For this review, take the finished solid that the model builds, in its own axes (mm). Give positions to 0.01 mm unless a question says otherwise; leave off trailing zeros. Loops run counter-clockwise (first coordinate to the right, second up) from the corner with the lowest first, then second, coordinate; pieces in that order, holes last. Notation, with made-up numbers: (-23.5, -3) -> (3.5, -3) arc R20 cw to (3.5, 14) -> close; hole circle Ø5 at (-4, -14.75). An arc over 180 degrees is marked (long way). Answer as CSV lines item,"result". Start each with the question number.
Item 1: Add section A-A on y = 10. State the section outline as (x, z) points, plus the area to 4 significant figures.
Item 2: The part is to be moulded in two halves that separate along Y. For faces 1 (the face through (-240, 61, 116)), 2 (the face through (-241.52, 109.14, 120.08)), say which applies: +Y half, -Y half, draft (parallel to the pull), parting line (faces both ways), or undercut.
Item 3: For L1, parallel to Y at x = -241.3, z = 10, list the stretches that pass through material, from the lowest coordinate up. Write a range as from..to.
Item 4: Add section B-B on z = 10. State the section outline as (x, y) points, plus the area to 3 significant figures.
Item 5: Add section C-C on z = 106.5. State the section outline as (x, y) points, plus the area to 3 significant figures.
```python
from build123d import *

# Parameters (mm, degrees)
SKETCH_1_W          = 236
SKETCH_1_H          = 126
EXTRUDE_1_DEPTH     = 3
SKETCH_2_R          = 2.25
CUT_EXTRUDE_1_DEPTH = 4
SKETCH_3_W          = 12
SKETCH_3_H          = 8
CUT_EXTRUDE_2_DEPTH = 4


with BuildPart() as part:
    # Эскиз1 → Бобышка-Вытянуть1 (new body)
    with BuildSketch(Plane.ZY.offset(240)):
        with Locations((118, 60)):
            Rectangle(SKETCH_1_W, SKETCH_1_H)
    extrude(amount=EXTRUDE_1_DEPTH)

    # Эскиз2 → Вырез-Вытянуть1 (cut, through all)
    with BuildSketch(Plane.ZY.offset(243)):
        with Locations((226, 110)):
            Circle(SKETCH_2_R)
        with Locations((118, 110)):
            Circle(SKETCH_2_R)
        with Locations((10, 110)):
            Circle(SKETCH_2_R)
        with Locations((226, 10)):
            Circle(SKETCH_2_R)
        with Locations((118, 10)):
            Circle(SKETCH_2_R)
        with Locations((10, 10)):
            Circle(SKETCH_2_R)
    extrude(amount=-CUT_EXTRUDE_1_DEPTH, mode=Mode.SUBTRACT)

    # Эскиз3 → Вырез-Вытянуть2 (cut, through all)
    with BuildSketch(Plane(origin=(-240, 0, 0), x_dir=(0, 0, -1), z_dir=(1, 0, 0))):
        with Locations((-103, 58.3)):
            Rectangle(SKETCH_3_W, SKETCH_3_H)
    extrude(amount=-CUT_EXTRUDE_2_DEPTH, mode=Mode.SUBTRACT)


solid = part.part
```
Computed values:
1,outline,"(-243, 0) -> (-240, 0) -> (-240, 7.75) -> (-243, 7.75) -> close; (-243, 12.25) -> (-240, 12.25) -> (-240, 115.75) -> (-243, 115.75) -> close; (-243, 120.25) -> (-240, 120.25) -> (-240, 223.75) -> (-243, 223.75) -> close; (-243, 228.25) -> (-240, 228.25) -> (-240, 236) -> (-243, 236) -> close"
1,area,"667.5 mm²"
2,face 1,"draft"
2,face 2,"undercut"
3,L1,"-3..7.75, 12.25..107.75, 112.25..123"
4,outline,"(-243, -3) -> (-240, -3) -> (-240, 7.75) -> (-243, 7.75) -> close; (-243, 12.25) -> (-240, 12.25) -> (-240, 107.75) -> (-243, 107.75) -> close; (-243, 112.25) -> (-240, 112.25) -> (-240, 123) -> (-243, 123) -> close"
4,area,"351 mm²"
5,outline,"(-243, -3) -> (-240, -3) -> (-240, 54.3) -> (-243, 54.3) -> close; (-243, 62.3) -> (-240, 62.3) -> (-240, 123) -> (-243, 123) -> close"
5,area,"354 mm²"
